```python
from build123d import *

# Parameters (mm, degrees)
EXTRUDE_1_DEPTH             = 10
EXTRUDE_2_REACH             = 34.619
SKETCH_2_R                  = 10
EXTRUDE_2_DIRECTION_2_DEPTH = 2
SKETCH_6_R                  = 1.65
SKETCH_6_W                  = 14.704506527
SKETCH_6_H                  = 8.520368268
CUT_EXTRUDE_2_DEPTH         = 43.983979574
FILLET_1_R                  = 1
FILLET_2_R                  = 0.5
EXTRUDE_3_DEPTH             = 8
EXTRUDE_4_DEPTH             = 55
SKETCH_9_W                  = 73
SKETCH_9_H                  = 45
CUT_EXTRUDE_3_DEPTH         = 13
SKETCH_10_W                 = 15
SKETCH_10_H                 = 20
CUT_EXTRUDE_4_DEPTH         = 13
SKETCH_11_W                 = 73
SKETCH_11_H                 = 45
CUT_EXTRUDE_6_DEPTH         = 13
SKETCH_12_W                 = 15
SKETCH_12_H                 = 45
SKETCH_12_W_2               = 10
EXTRUDE_5_DEPTH             = 5
FILLET_3_R                  = 3
SKETCH_14_R                 = 1.55
CUT_EXTRUDE_7_DEPTH         = 102.004950374


with BuildPart() as part:
    # 草图1 → 凸台-拉伸1 (new, symmetric)
    with BuildSketch(Plane.XY):
        with BuildLine():
            Line((-1.15, 3.987480407), (-1.15, 12))
            Line((-1.15, 12), (-4.15, 12))
            Line((-4.15, 12), (-4.15, 4.333301282))
            ThreePointArc((-4.15, 4.333301282), (-4.784308974, 3.620826928), (-5.297685557, 2.816829377))
            Line((-5.297685557, 2.816829377), (-8, -2.265484914))
            Line((-8, -2.265484914), (-8, -30))
            Line((-8, -30), (0, -30))
            Line((0, -30), (0, -8.485281374))
            Line((0, -8.485281374), (4.242640687, -4.242640687))
            ThreePointArc((4.242640687, -4.242640687), (5.999649956, 0.064810571), (4.15, 4.333301282))
            Line((4.15, 4.333301282), (4.15, 12))
            Line((4.15, 12), (1.15, 12))
            Line((1.15, 12), (1.15, 3.987480407))
            ThreePointArc((1.15, 3.987480407), (0, -4.15), (-1.15, 3.987480407))
        make_face()
    extrude(amount=EXTRUDE_1_DEPTH, both=True)

    # 凸台-拉伸2: up to this face of the body (flat: up to its plane)
    extrude_2_end = Plane(part.part.faces().sort_by_distance((-8, -16.132742457, 0))[0])
    # 草图2 → 凸台-拉伸2 (add, up to the picked face)
    with BuildSketch(Plane(origin=(0, 0, 0), x_dir=(0, 0, -1), z_dir=(1, 0, 0)), mode=Mode.PRIVATE) as extrude_2_sk1:
        with Locations((0, -30)):
            Circle(SKETCH_2_R)
    extrude_2_tool1 = split(extrude(extrude_2_sk1.sketch, amount=-EXTRUDE_2_REACH, mode=Mode.PRIVATE), bisect_by=extrude_2_end, keep=Keep.BOTH, mode=Mode.PRIVATE)
    add(extrude_2_tool1.solids().sort_by(Axis((0, -30, 0), (-1, 0, 0)))[0])

    # 草图2 → 凸台-拉伸2 direction 2 (add)
    with BuildSketch(Plane(origin=(0, 0, 0), x_dir=(0, 0, -1), z_dir=(1, 0, 0))):
        with Locations((0, -30)):
            Circle(SKETCH_2_R)
    extrude(amount=EXTRUDE_2_DIRECTION_2_DEPTH)

    # 草图6 → 切除-拉伸2 (cut, through all)
    with BuildSketch(Plane(origin=(4.15, 0, 0), x_dir=(0, 0, -1), z_dir=(1, 0, 0))):
        with Locations(Location((0, 9.5, 0), (0, 0, 90))):
            Circle(SKETCH_6_R)
        with Locations((-12.852253263, 11.760184134)):
            Rectangle(SKETCH_6_W, SKETCH_6_H)
        with Locations((12.852253263, 11.760184134)):
            Rectangle(SKETCH_6_W, SKETCH_6_H)
    extrude(amount=-CUT_EXTRUDE_2_DEPTH, mode=Mode.SUBTRACT)

    # 圆角1
    fillet_1_edges = [part.edges().sort_by_distance(p)[0] for p in [
        (2.65, 7.5, -10),
        (-2.65, 7.5, -10),
        (2.65, 7.5, 10),
        (-2.65, 7.5, 10),
        (2.65, 12, 5.5),
        (-2.65, 12, 5.5),
        (2.65, 12, -5.5),
        (-2.65, 12, -5.5),
    ]]
    fillet(fillet_1_edges, radius=FILLET_1_R)

    # 圆角2
    fillet_2_edges = [part.edges().sort_by_distance(p)[0] for p in [
        (-2.65, 7.5, 5.5),
        (2.65, 7.5, 5.5),
        (2.65, 7.5, -5.5),
        (-2.65, 7.5, -5.5),
    ]]
    fillet(fillet_2_edges, radius=FILLET_2_R)

    # 草图7 → 凸台-拉伸3 (add)
    with BuildSketch(Plane(origin=(2, 0, 0), x_dir=(0, 0, -1), z_dir=(1, 0, 0))):
        with BuildLine():
            Line((0, -20), (-22, -20))
            Line((-22, -20), (-22, -40))
            Line((-22, -40), (0, -40))
            ThreePointArc((0, -40), (10, -30), (0, -20))
        make_face()
    extrude(amount=EXTRUDE_3_DEPTH)

    # 草图8 → 凸台-拉伸4 (add)
    with BuildSketch(Plane.XY.offset(22)):
        Polygon((10, -20), (-26, -20), (-26, -40), (2, -40), (57, -40), (57, -20), align=None)
    extrude(amount=EXTRUDE_4_DEPTH)

    # 草图9 → 切除-拉伸3 (cut)
    with BuildSketch(Plane(origin=(0, -20, 0), x_dir=(1, 0, 0), z_dir=(0, 1, 0))):
        with Locations((15.5, -49.5)):
            Rectangle(SKETCH_9_W, SKETCH_9_H)
    extrude(amount=-CUT_EXTRUDE_3_DEPTH, mode=Mode.SUBTRACT)

    # 草图10 → 切除-拉伸4 (cut)
    with BuildSketch(Plane(origin=(0, 0, 22), x_dir=(-1, 0, 0), z_dir=(0, 0, -1))):
        with Locations((-17.5, -30)):
            Rectangle(SKETCH_10_W, SKETCH_10_H)
    extrude(amount=-CUT_EXTRUDE_4_DEPTH, mode=Mode.SUBTRACT)

    # 草图11 → 切除-拉伸6 (cut)
    with BuildSketch(Plane(origin=(0, -33, 0), x_dir=(1, 0, 0), z_dir=(0, 1, 0))):
        with Locations((15.5, -49.5)):
            Rectangle(SKETCH_11_W, SKETCH_11_H)
    extrude(amount=-CUT_EXTRUDE_6_DEPTH, mode=Mode.SUBTRACT)

    # 草图12 → 凸台-拉伸5 (add)
    with BuildSketch(Plane.XZ.offset(40)):
        with Locations((-13.5, 49.5)):
            Rectangle(SKETCH_12_W, SKETCH_12_H)
        with Locations((47, 49.5)):
            Rectangle(SKETCH_12_W_2, SKETCH_12_H)
    extrude(amount=-EXTRUDE_5_DEPTH)

    # 圆角3
    fillet_3_edges = [part.edges().sort_by_distance(p)[0] for p in [
        (-26, -30, 22),
        (57, -30, 22),
        (-26, -30, 77),
        (57, -30, 77),
        (10, -30, 27),
        (25, -30, 27),
    ]]
    fillet(fillet_3_edges, radius=FILLET_3_R)

    # 草图14 → 切除-拉伸7 (cut, through all)
    with BuildSketch(Plane(origin=(0, -20, 0), x_dir=(1, 0, 0), z_dir=(0, 1, 0))):
        with Locations(Location((-23, -25, 0), (0, 0, 270))):
            Circle(SKETCH_14_R)
        with Locations(Location((54, -25, 0), (0, 0, 270))):
            Circle(SKETCH_14_R)
        with Locations(Location((-23, -74, 0), (0, 0, 270))):
            Circle(SKETCH_14_R)
        with Locations(Location((54, -74, 0), (0, 0, 270))):
            Circle(SKETCH_14_R)
    extrude(amount=-CUT_EXTRUDE_7_DEPTH, mode=Mode.SUBTRACT)


solid = part.part
```
Work out the finished part from the listing and answer in its coordinate system (mm). A direction names the side the tool comes from. Coordinates: 2 decimals unless noted, no trailing zeros. Loops run counter-clockwise (first coordinate to the right, second up) from the corner with the lowest first, then second, coordinate; pieces in that order, holes last.
1) Section D-D (y = -24.5) is taken. Give the number of separate pieces and of enclosed holes in the cut face, plus the area to 3 significant figures.
Results:
separate pieces: 1
enclosed holes: 4
area: 1,600 mm2
2) Consider probe 1 along Z at (x, y) = (-7, -24); probe 2 along X at (y, z) = (-32, 66.5); probe 3 along X at (y, z) = (-24, 25). Determine where each line is inside the solid, lowest interval first.
Results:
probe 1: z = -10 to 10, 22 to 27, 72 to 77
probe 2: x = -26 to -21, 52 to 57
probe 3: x = -26 to -24.55, -21.45 to 9.83, 25.17 to 52.45, 55.55 to 57
3) Section C-C (x = -13) is taken. Give the vertices of the cut face in (y, z).
Results:
outline: (-40, 22) - (-20, 22) - (-20, 27) - (-35, 27) - (-35, 72) - (-20, 72) - (-20, 77) - (-40, 77) - close
4) For faces 1 (the flat face through (-6, -38, 49)), 2 (the flat face through (15, -30, 72)), 3 (the flat face through (-4.15, 7, 0)), 4 (the cylindrical face through (-2.629, 11.024, -0.632)), 5 (the flat face through (-3, 7.5, 8)), determine the directions among +Z, -Z, +X, -X, +Y, -Y from which every point of the face is accessible in a straight line to the end or side of a thin tool.
Results:
face 1: +Y, -Y
face 2: +Y
face 3: +Z, -Z, -X, +Y
face 4: +X, -X
face 5: +Z, +X, -X, +Y
5) Flat-ended cylindrical pins translate along their axes: pin 1 (7 mm diameter, centred on x = -0.5, y = -12, fed in from +Z); pin 2 (3.5 mm diameter, centred on x = -2, y = 9.5, fed in from -Z); pin 3 (12 mm diameter, centred on x = -11, z = 7, fed in from -Y). Find the tip coordinate at first contact, or state that the pin passes through.
Results:
pin 1: stops at z = 10
pin 2: stops at z = -5.57
pin 3: stops at y = -39.84
6) Section B-B (x = 39.5) is taken. Give the vertices of the cut face in (y, z).
Results:
outline: (-40, 22) - (-20, 22) - (-20, 27) - (-40, 27) - close; (-40, 72) - (-20, 72) - (-20, 77) - (-40, 77) - close
7) Section A-A (z = 47) is taken. Give the vertices of the cut face in (x, y), plus the area to 3 significant figures.
Results:
outline: (-26, -40) - (-6, -40) - (-6, -35) - (-21, -35) - (-21, -20) - (-26, -20) - close; (42, -40) - (57, -40) - (57, -20) - (52, -20) - (52, -35) - (42, -35) - close
area: 325 mm2
8) For a pull along Z with two mould halves and no side action, classify faces 6 (the cylindrical face through (2.671, 11.024, -0.632)), 7 (the cylindrical face through (56.1, -29.86, 76.14)), 8 (the flat face through (3, 7.5, -7)) as +Z half, -Z half, draft (parallel to the pull), parting line (faces both ways), or undercut.
Results:
face 6: undercut
face 7: +Z half
face 8: draft
